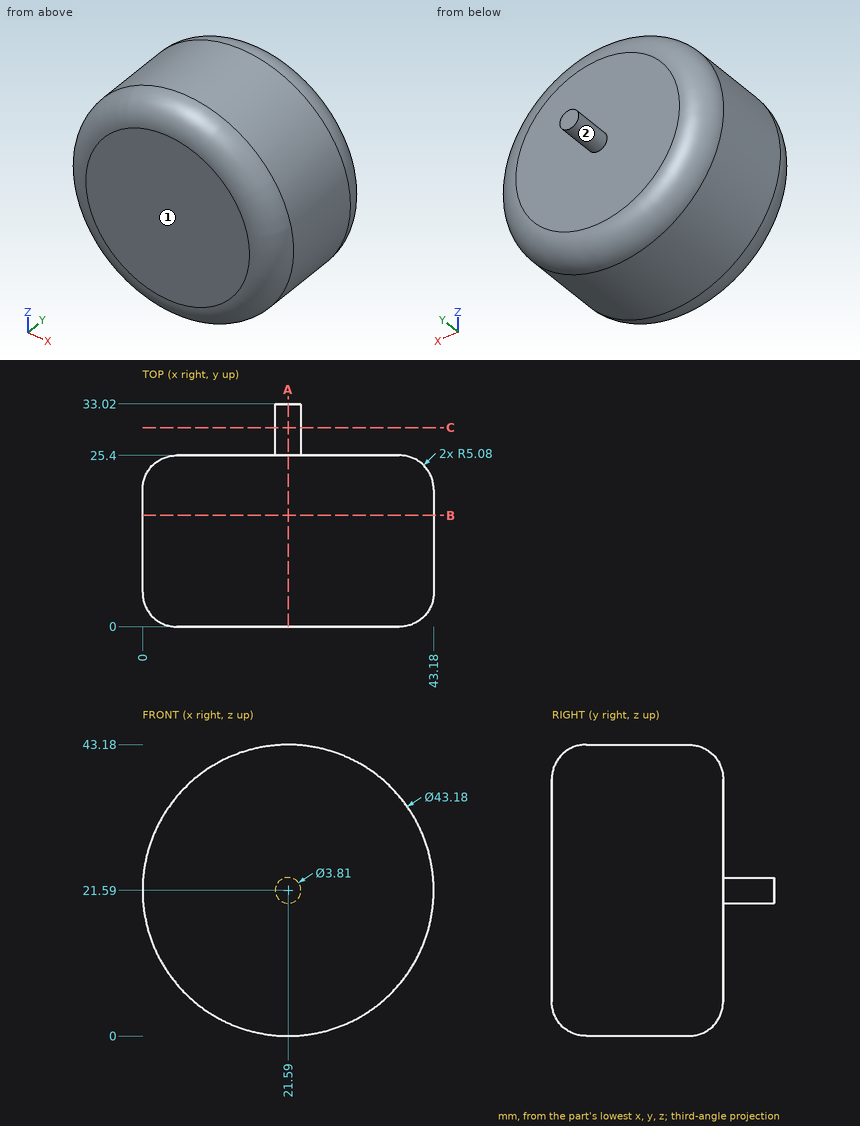
Study the drawing (mm; zero at the part's minimum x, y, z) and answer. A direction names the side the tool comes from. Round coordinates to 2 decimals unless told otherwise and drop trailing zeros. Write each loop counter-clockwise with the first axis right and the second up, starting at its lowest first coordinate (ties: lowest second). Pieces come first, ordered by that corner, then holes.
1) A cutting plane is placed at C-C on y = 29.5. Determine the outline of the cut face in (x, z) (3 decimals), and give its area (3 significant figures).
2) Which of the six approach directions +Z, -Z, +X, -X, +Y, -Y give full straight-line access (tool end or side, diameter ignored) to the marked faces 1 and 2?
3) Consider probe 1 along Y at (x, z) = (24, 26); probe 2 along Z at (x, y) = (21.5, 10.5); probe 3 along X at (y, z) = (17, 21). Determine where each line is inside the solid, lowest interval first.
4) A cutting plane is placed at A-A on x = 21.59. Determine the outline of the cut face in (y, z) (3 decimals), and give its area (3 significant figures).
5) A cutting plane is placed at B-B on y = 16.5. Determine the outline of the cut face in (x, z).
6) Flat-ended cylindrical pins translate along their axes: P1, Ø5, axis at x = 10.5, y = 22, coming from the +Z side; P2, Ø12, axis at x = 9, z = 37.5, coming from the +Y side; P3, Ø5, axis at x = 32, y = 5, coming from the +Z side. Find the tip coordinate at first contact, or state that the pin passes through.
Entries:
1. outline: circle Ø3.81 at (21.59, 21.59)
1. area: 11.4 mm2
2. face 1: +Z, -Z, +X, -X, -Y
2. face 2: +Y
3. probe 1: y = 0 to 25.4
3. probe 2: z = 0 to 43.18
3. probe 3: x = 0.01 to 43.17
4. outline: (0, 5.08) arc R5.08 ccw to (5.08, 0) - (20.32, 0) arc R5.08 ccw to (25.4, 5.08) - (25.4, 19.685) - (33.02, 19.685) - (33.02, 23.495) - (25.4, 23.495) - (25.4, 38.1) arc R5.08 ccw to (20.32, 43.18) - (5.08, 43.18) arc R5.08 ccw to (0, 38.1) - close
4. area: 1,100 mm2
5. outline: circle Ø43.18 at (21.59, 21.59)
6. P1: stops at z = 41.26
6. P2: stops at y = 25.4
6. P3: stops at z = 41.68
